Job drawing, mm, ordinate dimensions from the low corner. One solid piece. Coordinates: 2 decimals unless noted, no trailing zeros. Loops run counter-clockwise (first coordinate to the right, second up) from the corner with the lowest first, then second, coordinate; pieces in that order, holes last. Notation, with made-up numbers: (34.5, 18.25) -> (93.5, 18.25) arc R17 ccw to (93.5, 39.25) -> close; hole circle Ø10 at (8.5, -17). An arc over 180 degrees is marked (long way). Use one line per item in the form item = value. Start each with the question number.
(1) Drill centre lines: L1, parallel to X at y = 1, z = 4.25; L2, parallel to Y at x = 28, z = 1.25; L3, parallel to Z at x = 193.5, y = 1.5 (1 decimal). Where is each one in solid material? Low to high. Write a range as [from, to].
(2) Band-saw the part on B-B on z = 4.5. Give the cut face in (x, y).
(3) Pin check, flat tips, straight feed: P1, Ø3, axis at y = 2, z = 4, coming from the -X side; P2, Ø3, axis at x = 156, y = 5, coming from the +Z side (1 decimal); P3, Ø1.5, axis at x = 164.5, z = 4, coming from the +Y side. Stop position of each tip, or through.
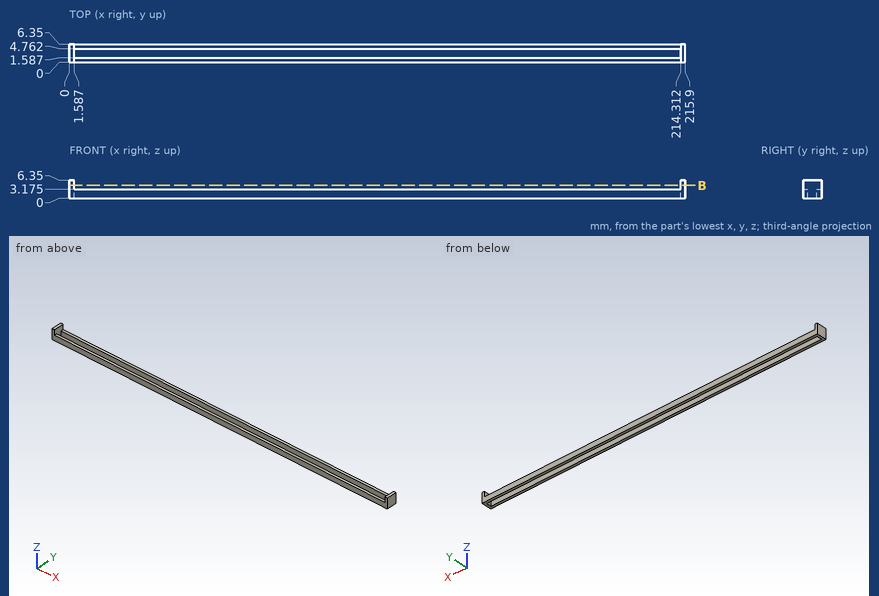
A:
q1.L1 = [0, 1.59], [214.31, 215.9]
q1.L2 = [0, 1.59], [4.76, 6.35]
q1.L3 = [0, 3.2]
q2.outline = (0, 0) -> (1.59, 0) -> (1.59, 6.35) -> (0, 6.35) -> close; (214.31, 0) -> (215.9, 0) -> (215.9, 6.35) -> (214.31, 6.35) -> close
q3.P1 = 0
q3.P2 = 3.2
q3.P3 = through
